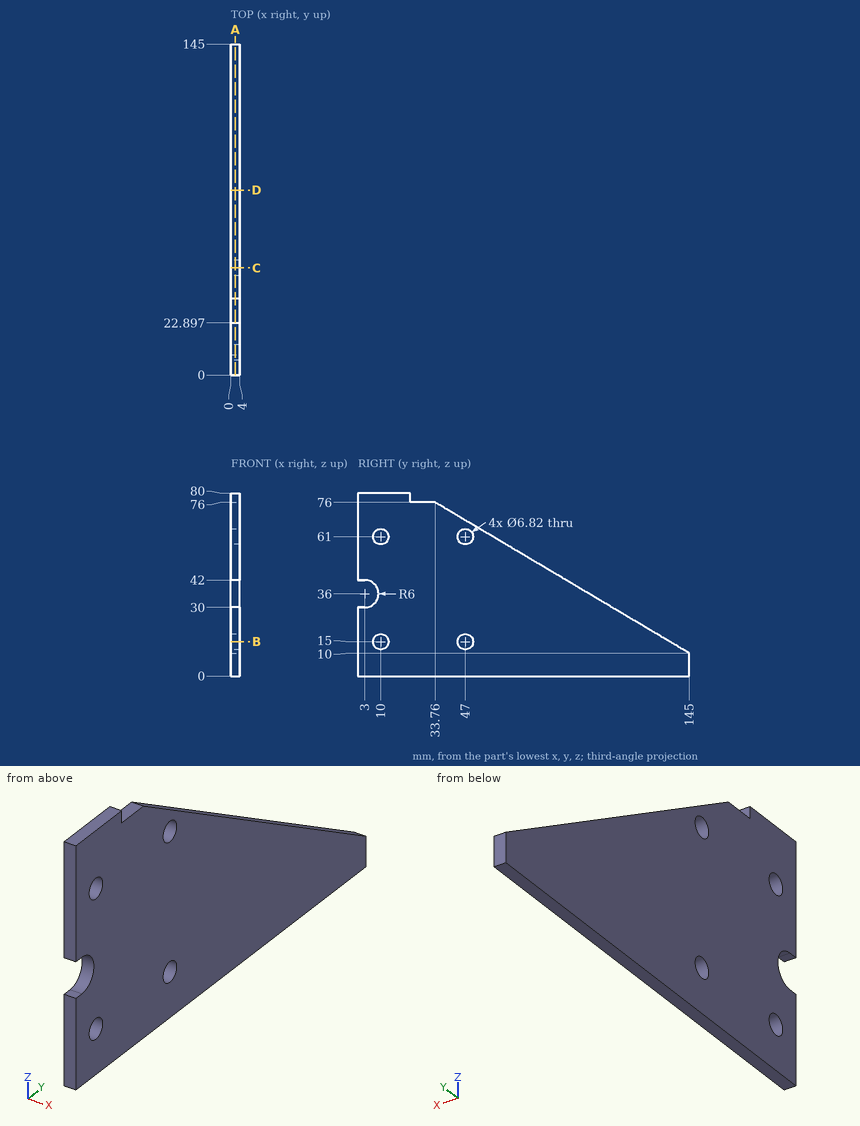
Design review of the part shown in the three views and the two pictorial views. Dimensions are in mm from the part's minimum x, y and z. Round coordinates to 2 decimals unless told otherwise and drop trailing zeros. Order: outer loops, then holes, each group sorted by start corner. A loop starts at its lowest first (then second) coordinate and runs counter-clockwise, first axis right, second up.
Item 1: Add section B-B, the plane z = 15. State the section outline as (x, y) points, and give its area (3 significant figures).
Working result:
outline: (0, 0) - (4, 0) - (4, 6.59) - (0, 6.59) - close; (0, 13.41) - (4, 13.41) - (4, 43.59) - (0, 43.59) - close; (0, 50.41) - (4, 50.41) - (4, 136.57) - (0, 136.57) - close
area: 492 mm2
Item 2: Add section A-A, the plane x = 2. State the section outline as (y, z) points, and give its area (3 significant figures).
Working result:
outline: (0, 0) - (145, 0) - (145, 10) - (33.76, 76) - (22.9, 76) - (22.9, 80) - (0, 80) - (0, 42) - (3, 42) arc R6 cw to (3, 30) - (0, 30) - close; hole circle Ø6.82 at (10, 15); hole circle Ø6.82 at (10, 61); hole circle Ø6.82 at (47, 15); hole circle Ø6.82 at (47, 61)
area: 7,200 mm2
Item 3: Add section D-D, the plane y = 81. State the section outline as (x, z) points.
Working result:
outline: (0, 0) - (4, 0) - (4, 47.97) - (0, 47.97) - close
Item 4: To check wall thickness, follow probe 1 along Z at (x, y) = (2.75, 12); probe 2 along Y at (x, z) = (3.2, 61); probe 3 along Y at (x, z) = (1.1, 15) (1 decimal). State the ranges of each line that lie inside material, in increasing order.
Working result:
probe 1: z = 0 to 12.24, 17.76 to 58.24, 63.76 to 80
probe 2: y = 0 to 6.59, 13.41 to 43.59, 50.41 to 59.04
probe 3: y = 0 to 6.6, 13.4 to 43.6, 50.4 to 136.6
Item 5: Add section C-C, the plane y = 47. State the section outline as (x, z) points (1 decimal), and give its area (3 significant figures).
Working result:
outline: (0, 0) - (4, 0) - (4, 11.6) - (0, 11.6) - close; (0, 18.4) - (4, 18.4) - (4, 57.6) - (0, 57.6) - close; (0, 64.4) - (4, 64.4) - (4, 68.1) - (0, 68.1) - close
area: 218 mm2
Item 6: For pin 1 (1.2 mm diameter, centred on x = 2.5, z = 78, fed in from +Y), flat-tipped, find the tip position at first contact; note if it passes through.
Working result:
pin 1: stops at y = 22.9
